Read the model definition and answer for the solid it produces. Units are mm, in the model's axes. A direction names the side the tool comes from. Coordinates: 2 decimals unless noted, no trailing zeros. Order: outer loops, then holes, each group sorted by start corner. A loop starts at its lowest first (then second) coordinate and runs counter-clockwise, first axis right, second up. Notation, with made-up numbers: (5, 6.5) - (42, 6.5) arc R26 cw to (42, 33.5) - close; hole circle Ø7 at (48, 76). An arc over 180 degrees is marked (long way). Write item = value, one per line.
Autodesk Inventor part; units mm, degrees
ref_plane "Work Plane2" through (-14.1414, -14.1414, 86.5) normal (0, 0, -1) x (0, 1, 0)
ref_plane "YZ Plane" through (0, 0, 0) normal (1, 0, 0) x (0, 1, 0)
ref_plane "XZ Plane" through (0, 0, 0) normal (0, 1, 0) x (-1, 0, 0)
ref_plane "Work Plane1" through (0, 0, 0) normal (0, 0, 1) x (1, 0, 0)
sketch "Sketch1" plane through (0, 0, 0) normal (0, 0, 1) x (1, 0, 0)
  line L0 (-40, -40) -> (40, -40)
  line L1 (40, -40) -> (40, 40)
  line L2 (40, 40) -> (-40, 40)
  line L3 (-40, 40) -> (-40, -40)
  line L4 (-40, -40) -> (40, 40) construction
  line L5 (40, -40) -> (-40, 40) construction
  point P0 (0, 0)
  dimension "d0" = 80
extrude "Extrusion1" add sketch "Sketch1" along normal blind 2
ref_plane "Work Plane2" through (-14.1414, -14.1414, 86.5) normal (0, 0, -1) x (0, 1, 0)
sketch "Sketch2" plane through (0, 0, 2) normal (0, 0, 1) x (1, 0, 0)
  circle A0 centre (0, 0) radius 42.5 construction
  circle A1 centre (30.052, 30.052) radius 4
  line L0 (0, 0) -> (30.052, 30.052) construction
  line L1 (-40, -40) -> (40, -40)
  circle A2 centre (-30.052, 30.052) radius 4
  circle A3 centre (-30.052, -30.052) radius 4
  circle A4 centre (30.052, -30.052) radius 4
  dimension "d3" = 85
  dimension "d4" = 45
  dimension "d5" = 8
  dimension "d8" = 360
extrude "Extrusion2" add sketch "Sketch2" along normal up to surface (84.5 mm away)
ref_plane "Work Plane3" through (0, 0, 86.5) normal (0, 0, -1) x (1, 0, 0)
sketch "Sketch3" plane through (0, 0, 86.5) normal (0, 0, -1) x (1, 0, 0)
  line L0 (40, -40) -> (-40, -40)
  circle A0 centre (30.052, -30.052) radius 4
  circle A1 centre (-30.052, 30.052) radius 4
  circle A2 centre (30.052, 30.052) radius 4
  circle A3 centre (-30.052, -30.052) radius 4
  line L1 (40, -40) -> (-40, -40)
  line L2 (-40, -40) -> (-40, 40)
  line L3 (-40, 40) -> (40, 40)
  line L4 (40, 40) -> (40, -40)
  circle A4 centre (0, 0) radius 12.5
  circle A5 centre (-17.5, 0) radius 2
  circle A6 centre (0, 17.5) radius 2
  circle A7 centre (0, -17.5) radius 2
  circle A8 centre (17.5, 0) radius 2
  circle A9 centre (0, 0) radius 20.85
  circle A10 centre (0, 0) radius 4
  point P0 (0, 0)
  point P1 (40, -40)
  point P2 (-40, -40)
extrude "Extrusion3" add sketch "Sketch3" along normal blind 2 contours L0 L2 L3 L4 | A4 | A9
sketch "Sketch4" plane through (0, 0, 86.5) normal (0, 0, -1) x (1, 0, 0)
  line L0 (40, -40) -> (40, 40)
  line L1 (-40, -40) -> (40, -40)
  line L2 (-40, 40) -> (-40, -40)
  line L3 (40, 40) -> (-40, 40)
  circle A0 centre (0, 0) radius 12.5
  line L4 (40, -40) -> (40, 40)
  line L5 (-40, -40) -> (40, -40)
  line L6 (-40, 40) -> (-40, -40)
  line L7 (40, 40) -> (-40, 40)
  circle A1 centre (0, 0) radius 4
  circle A2 centre (0, 17.5) radius 2
  circle A3 centre (0, -17.5) radius 2
  circle A4 centre (-17.5, 0) radius 2
  circle A5 centre (17.5, 0) radius 2
  point P0 (0, 0)
extrude "Extrusion4" add sketch "Sketch4" against normal blind 2 contours L1 L2 L3 L0
properties part number "motor to gearbox flange"
1) The part is cut by section B-B (x = -23). Determine the outline of the cut face in (y, z).
Returned:
outline = (-40, 0) - (40, 0) - (40, 2) - (-40, 2) - close; (-40, 84.5) - (40, 84.5) - (40, 88.5) - (-40, 88.5) - close
2) The part is cut by section A-A (y = 17.5). Determine the outline of the cut face in (x, z), and give its area (3 significant figures).
Returned:
outline = (-40, 0) - (40, 0) - (40, 2) - (-40, 2) - close; (-40, 84.5) - (-2, 84.5) - (-2, 88.5) - (-40, 88.5) - close; (2, 84.5) - (40, 84.5) - (40, 88.5) - (2, 88.5) - close
area = 464 mm^2
3) Flat-ended cylindrical pins translate along their axes: pin 1 Ø12 at (x, z) = (18.5, 36) entering from -Y; pin 2 Ø6.5 at (x, y) = (0, 0) entering from +Z; pin 3 Ø12.5 at (x, y) = (-0.5, -5.5) entering from +Z; pin 4 Ø2 at (x, z) = (-28.5, 19.5) entering from +Y. Find the tip coordinate at first contact, or state that the pin passes through.
Returned:
pin_1 = through
pin_2 = 2
pin_3 = 86.5
pin_4 = 34.01
4) Determine the mould class of faces 1 (the face through (32.202, -33.425, 42.672)), 2 (the face through (-9, -9, 88.5)), 3 (the face through (33.75, 31.58, 42.67)), 4 (the face through (15.9, 1.2, 86.5)) for opening direction Z: pulls with the +Z half, pulls with the -Z half, needs draft (parallel to the pull), parting line crosses it, or undercut.
Returned:
face_1 = undercut
face_2 = pulls with the +Z half
face_3 = undercut
face_4 = needs draft
5) For faces 5 (the face through (-40, -1, 86)), 6 (the face through (-0.867, -3.905, 85.514)), 7 (the face through (-26.237, -31.253, 42.672)), determine the directions among +Z, -Z, +X, -X, +Y, -Y from which every point of the face is accessible in a straight line to the end or side of a thin tool.
Returned:
face_5 = +Z, -Z, -X, +Y, -Y
face_6 = +Z
face_7 = none
6) The part is cut by section C-C (x = 0). Determine the outline of the cut face in (y, z).
Returned:
outline = (-40, 0) - (40, 0) - (40, 2) - (-40, 2) - close; (-40, 84.5) - (-19.5, 84.5) - (-19.5, 88.5) - (-40, 88.5) - close; (-15.5, 84.5) - (-4, 84.5) - (-4, 86.5) - (-12.5, 86.5) - (-12.5, 88.5) - (-15.5, 88.5) - close; (4, 84.5) - (15.5, 84.5) - (15.5, 88.5) - (12.5, 88.5) - (12.5, 86.5) - (4, 86.5) - close; (19.5, 84.5) - (40, 84.5) - (40, 88.5) - (19.5, 88.5) - close
7) Straight lines are drawn through the part: line 1 along X through (y, z) = (0, 85.8); line 2 along X through (y, z) = (0, 87); line 3 along Y through (x, z) = (-30.5, 37.5). For each, find the intervals that lie inside material, in ascending order. Write a range as from..to.
Returned:
line_1 = -40..-19.5, -15.5..-4, 4..15.5, 19.5..40
line_2 = -40..-19.5, -15.5..-12.5, 12.5..15.5, 19.5..40
line_3 = -34.03..-26.08, 26.08..34.03
8) The part is cut by section D-D (x = 31). Determine the outline of the cut face in (y, z), and give its area (3 significant figures).
Returned:
outline = (-40, 0) - (40, 0) - (40, 2) - (33.94, 2) - (33.94, 84.5) - (40, 84.5) - (40, 88.5) - (-40, 88.5) - (-40, 84.5) - (-33.94, 84.5) - (-33.94, 2) - (-40, 2) - close; hole (-26.17, 2) - (26.17, 2) - (26.17, 84.5) - (-26.17, 84.5) - close
area = 1,760 mm^2
